The figure shows three views and two pictorial views of one solid part (mm, origin at its lowest corner). Answer the questions. Coordinates: 2 decimals unless noted, no trailing zeros. Order: outer loops, then holes, each group sorted by start corner. A loop starts at its lowest first (then second) coordinate and runs counter-clockwise, first axis right, second up.
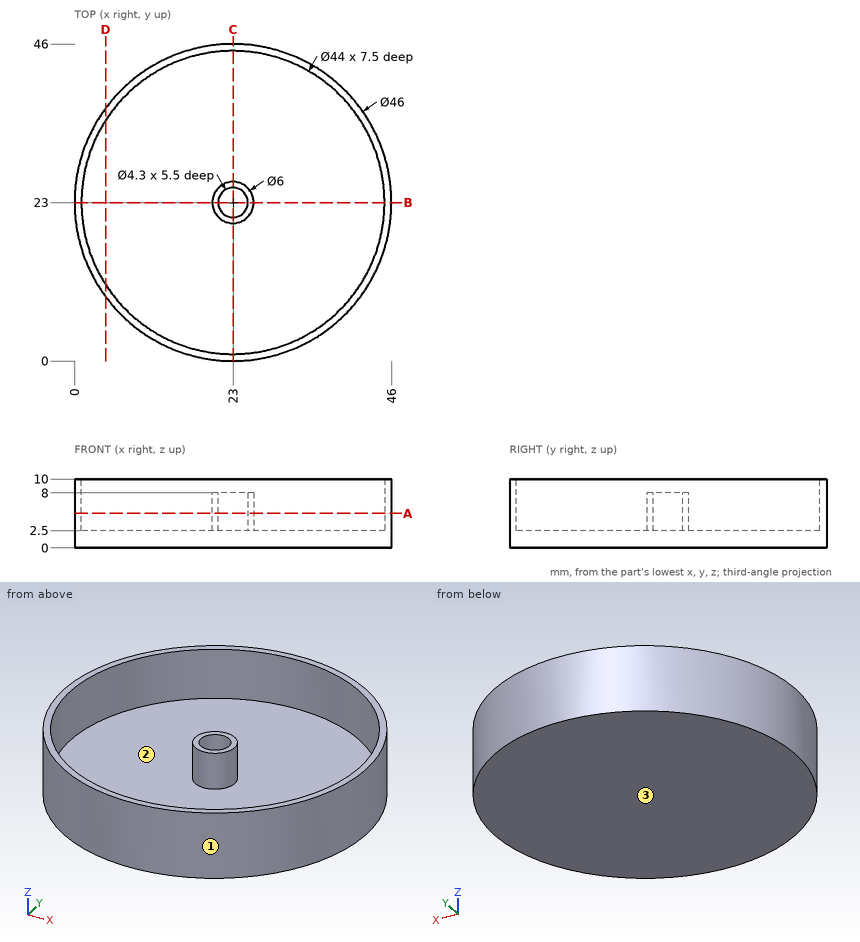
1) The mould has two halves that part along Y. Classify the marked faces 1, 2 and 3: released by +Y, released by -Y, zero draft, split by the parting line, or undercut.
2) Straight lines are drawn through the part: probe 1 along Y at (x, z) = (23, 6.2); probe 2 along Y at (x, z) = (22, 6); probe 3 along Z at (x, y) = (10.5, 20). For each, find the intervals that lie inside material, in ascending order.
3) A cutting plane is placed at B-B, the plane y = 23. Write down the section's boundary in (x, z), plus the area to 3 significant figures.
4) Each of these flat-tipped pins is pushed along its axis until it touches: P1, Ø5, axis at y = 13.5, z = 4, coming from the -X side; P2, Ø6, axis at y = 30, z = 7.5, coming from the -X side; P3, Ø6, axis at x = 34.5, z = 3.5, coming from the -Y side. Where does it stop, or does it pass through?
5) A cutting plane is placed at A-A, the plane z = 5. Write down the section's boundary in (x, y).
6) A cutting plane is placed at D-D, the plane x = 4.5. Write down the section's boundary in (y, z), plus the area to 3 significant figures.
Working result:
1. face 1: split by the parting line
1. face 2: undercut
1. face 3: zero draft
2. probe 1: y = 0 to 1, 20 to 20.85, 25.15 to 26, 45 to 46
2. probe 2: y = 0.02 to 1.02, 20.17 to 21.1, 24.9 to 25.83, 44.98 to 45.98
2. probe 3: z = 0 to 2.5
3. outline: (0, 0) - (46, 0) - (46, 10) - (45, 10) - (45, 2.5) - (26, 2.5) - (26, 8) - (25.15, 8) - (25.15, 2.5) - (20.85, 2.5) - (20.85, 8) - (20, 8) - (20, 2.5) - (1, 2.5) - (1, 10) - (0, 10) - close
3. area: 139 mm2
4. P1: stops at x = 1.09
4. P2: stops at x = 0.35
4. P3: stops at y = 1.63
5. outline: circle Ø46 at (23, 23); circle Ø6 at (23, 23); hole circle Ø44 at (23, 23); hole circle Ø4.3 at (23, 23)
6. outline: (9.33, 0) - (36.67, 0) - (36.67, 10) - (34.91, 10) - (34.91, 2.5) - (11.09, 2.5) - (11.09, 10) - (9.33, 10) - close
6. area: 94.7 mm2
